Can you work these out from the drawing? Everything is in mm from the part's minimum corner. Coordinates: 2 decimals unless noted, no trailing zeros. Write each loop counter-clockwise with the first axis right and the second up, starting at its lowest first coordinate (ties: lowest second). Pieces come first, ordered by that corner, then holes. Notation, with made-up numbers: (-19, 40.5) -> (29, 40.5) arc R17 cw to (29, 70.5) -> close; hole circle Ø11 at (28.25, 80). An arc over 180 degrees is marked (long way). Answer as CSV lines item,"result". Start each with the question number.
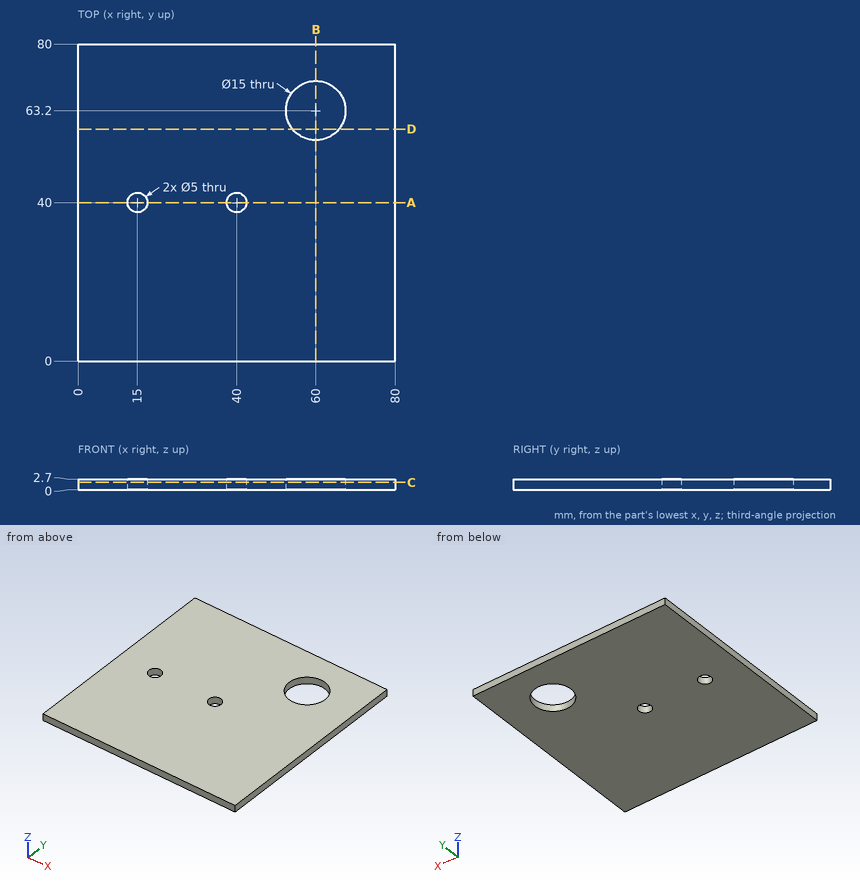
Q1. I need wall thicknesses on L1, parallel to Y at x = 40, z = 0.9; L2, parallel to Y at x = 60, z = 0.9; L3, parallel to X at y = 66, z = 0.95. Which ranges of each line are inside material? Lowest first, please.
Q2. Imagine slicing it at B-B (x = 60). Write out the boundary of the cut face in (y, z).
Q3. Imagine slicing it at D-D (y = 58.5). Write out the boundary of the cut face in (x, z).
Q4. Imagine slicing it at C-C (z = 1.85). Write out the boundary of the cut face in (x, y).
Q5. For pin 1 (3 mm diameter, centred on x = 15, y = 40, fed in from +Z), with a flat end and sliding along its axis, tell me the tip position at first contact or that it passes through.
Q6. Imagine slicing it at A-A (y = 40). Write out the boundary of the cut face in (x, z), then the cut area to 3 significant figures.
Entries:
1,L1,"0 to 37.5, 42.5 to 80"
1,L2,"0 to 55.7, 70.7 to 80"
1,L3,"0 to 53.04, 66.96 to 80"
2,outline,"(0, 0) -> (55.7, 0) -> (55.7, 2.7) -> (0, 2.7) -> close; (70.7, 0) -> (80, 0) -> (80, 2.7) -> (70.7, 2.7) -> close"
3,outline,"(0, 0) -> (54.16, 0) -> (54.16, 2.7) -> (0, 2.7) -> close; (65.84, 0) -> (80, 0) -> (80, 2.7) -> (65.84, 2.7) -> close"
4,outline,"(0, 0) -> (80, 0) -> (80, 80) -> (0, 80) -> close; hole circle Ø5 at (15, 40); hole circle Ø5 at (40, 40); hole circle Ø15 at (60, 63.2)"
5,pin 1,"through"
6,outline,"(0, 0) -> (12.5, 0) -> (12.5, 2.7) -> (0, 2.7) -> close; (17.5, 0) -> (37.5, 0) -> (37.5, 2.7) -> (17.5, 2.7) -> close; (42.5, 0) -> (80, 0) -> (80, 2.7) -> (42.5, 2.7) -> close"
6,area,"189 mm2"
